from build123d import *

# Parameters (mm, degrees)
EXTRUDE_1_OUTLINE_R = 1.5
EXTRUDE_1_DEPTH     = 3
EXTRUDE_2_DEPTH     = 25
EXTRUDE_3_DEPTH     = 3
EXTRUDE_4_REACH     = 147.278
FILLET_1_R          = 3
SKETCH_5_R          = 1.5
CUT_EXTRUDE_3_DEPTH = 15
SKETCH_6_R          = 126.976740186
SKETCH_6_R_2        = 100
CUT_EXTRUDE_4_DEPTH = 30
SKETCH_8_W          = 28.33895888
SKETCH_8_H          = 14.242713356
CUT_EXTRUDE_5_DEPTH = 5


# Read off the part's stored shape, not the designer's step: 填料-伸長1
with BuildPart() as part:
    # 填料-伸長1 outline → 填料-伸長1 (new body)
    with BuildSketch(Plane.XZ.offset(-131.641882403)):
        with BuildLine():
            ThreePointArc((-105.458191259, 52.468420543), (-108.501205852, 56.151510861), (-113.143070085, 55.020940854))
            Line((-113.143070085, 55.020940854), (-129.654103506, 38.071506203))
            ThreePointArc((-129.654103506, 38.071506203), (-130.77342938, 33.752171981), (-127.62304878, 30.592323786))
            Line((-127.62304878, 30.592323786), (-107.96955265, 30.592323786))
            ThreePointArc((-107.96955265, 30.592323786), (-104.412306977, 32.020558846), (-103.246421534, 35.67221098))
            Line((-103.246421534, 35.67221098), (-105.458191259, 52.468420543))
        make_face()
        with Locations((-126.430709133, 34.931485706)):
            Circle(EXTRUDE_1_OUTLINE_R, mode=Mode.SUBTRACT)
        with Locations((-107.707905988, 35.084710794)):
            Circle(EXTRUDE_1_OUTLINE_R, mode=Mode.SUBTRACT)
        with Locations((-109.919675712, 51.880920357)):
            Circle(EXTRUDE_1_OUTLINE_R, mode=Mode.SUBTRACT)
    extrude(amount=EXTRUDE_1_DEPTH)

    # 草圖2 → 填料-伸長2 (add)
    with BuildSketch(Plane.XZ.offset(-128.641882403)):
        Polygon((-104.786745972, 47.369455849), (-124.786745972, 47.369455849), (-124.786745972, 44.369455849), (-104.786745972, 44.369455849), (-104.391697962, 44.369455849), align=None)
    extrude(amount=EXTRUDE_2_DEPTH)

    # 草圖3 → 填料-伸長3 (add)
    with BuildSketch(Plane(origin=(0, 128.641882403, 0), x_dir=(1, 0, 0), z_dir=(0, 1, 0))):
        Polygon((-124.786745972, -47.369455849), (-120.596647578, -47.369455849), (-123.519051852, -44.369455849), (-124.786745972, -44.369455849), align=None)
    extrude(amount=EXTRUDE_3_DEPTH)

    # 填料-伸長4: up to this face of the body (flat: up to its plane)
    extrude_4_end = Plane(part.part.faces().sort_by_distance((-115.187288505, 131.641882403, 40.896845269))[0])
    # 草圖4 → 填料-伸長4 (add, up to the picked face)
    with BuildSketch(Plane.XZ.offset(-103.641882403), mode=Mode.PRIVATE) as extrude_4_sk1:
        with BuildLine():
            Line((-104.786745972, 47.369455849), (-103.657869092, 38.796749367))
            Line((-103.657869092, 38.796749367), (-128.657869092, 38.796749367))
            ThreePointArc((-128.657869092, 38.796749367), (-125.290449125, 43.179472861), (-121.686031693, 47.369455849))
            Line((-121.686031693, 47.369455849), (-104.786745972, 47.369455849))
        make_face()
    extrude_4_tool1 = split(extrude(extrude_4_sk1.sketch, amount=-EXTRUDE_4_REACH, mode=Mode.PRIVATE), bisect_by=extrude_4_end, keep=Keep.BOTH, mode=Mode.PRIVATE)
    add(extrude_4_tool1.solids().sort_by(Axis((-114.856202, 103.641882, 42.808825), (0, 1, 0)))[0])

    # 圓角1
    # the kernel refuses this fillet: 3 mm, written as the material it takes off along each edge
    with BuildSketch(Plane(origin=(-128.657869092, 88.125757689, 38.796749367), x_dir=(1, 0, 0), z_dir=(0, 1, 0))) as fillet_1_piece_1:
        with BuildLine():
            CenterArc((6.112644238, -3), FILLET_1_R, 90, 129.509532044)
            ThreePointArc((3.798087984, -4.90861975), (1.860953441, -2.483782776), (0, 0))
            Line((0, 0), (6.112644238, 0))
        make_face()
    extrude(amount=40.516124714, mode=Mode.SUBTRACT)
    with BuildSketch(Plane(origin=(-128.657869092, 88.125757689, 38.796749367), x_dir=(1, 0, 0), z_dir=(0, 1, 0))) as fillet_1_piece_2_section:
        with BuildLine():
            CenterArc((6.112644238, -3), FILLET_1_R, 90, 129.509532044)
            ThreePointArc((3.798087984, -4.90861975), (1.860953441, -2.483782776), (0, 0))
            Line((0, 0), (6.112644238, 0))
        make_face()
    fillet_1_piece_2 = extrude(amount=56.032249428, mode=Mode.PRIVATE)
    fillet_1_piece_2 = split(fillet_1_piece_2, bisect_by=Plane(origin=(-126.052723455, 130.141882403, 41.768510156), z_dir=(-0.7163098605374205, 0, 0.6977823326058501)), keep=Keep.TOP, mode=Mode.PRIVATE)
    add(fillet_1_piece_2, mode=Mode.SUBTRACT)
    with BuildSketch(Plane(origin=(-103.657869092, 95.089515631, 38.796749367), x_dir=(-0.13055559688671156, 0, 0.9914409897323968), z_dir=(0, 1, 0))) as fillet_1_piece_3:
        with BuildLine():
            CenterArc((FILLET_1_R * 1.14031556955, -FILLET_1_R), FILLET_1_R, 90, 97.501699304)
            Line((FILLET_1_R * 0.148874579822, -FILLET_1_R * 1.13055559689), (0, 0))
            Line((0, 0), (FILLET_1_R * 1.14031556955, 0))
        make_face()
    extrude(amount=33.552366772, mode=Mode.SUBTRACT)

    # 草圖5 → 除料-伸長3 (cut)
    with BuildSketch(Plane.XZ.offset(-103.641882403)):
        with Locations(Location((-106.94667544, 41.72393279, 0), (0, 0, 270))):
            Circle(SKETCH_5_R)
        with Locations(Location((-122.44667544, 41.72393279, 0), (0, 0, 270))):
            Circle(SKETCH_5_R)
    extrude(amount=-CUT_EXTRUDE_3_DEPTH, mode=Mode.SUBTRACT)

    # 草圖6 → 除料-伸長4 (cut)
    with BuildSketch(Plane.XZ.offset(-103.641882403)):
        with Locations((-47.707905988, -19.915289206)):
            Circle(SKETCH_6_R)
        with Locations((-47.707905988, -19.915289206)):
            Circle(SKETCH_6_R_2, mode=Mode.SUBTRACT)
    extrude(amount=-CUT_EXTRUDE_4_DEPTH, mode=Mode.SUBTRACT)

    # 草圖8 → 除料-伸長5 (cut)
    with BuildSketch(Plane.XZ.offset(-103.641882403)):
        with Locations((-114.972608674, 43.454782353)):
            Rectangle(SKETCH_8_W, SKETCH_8_H)
    extrude(amount=-CUT_EXTRUDE_5_DEPTH, mode=Mode.SUBTRACT)


solid = part.part
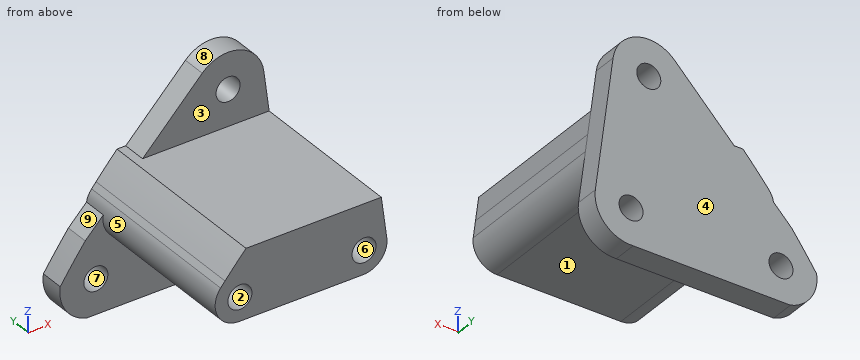
Input: part model. Units: mm. Frame: model coordinates. Face numbers are marked on the shaded views. A direction names the side the tool comes from. Round coordinates to 2 decimals unless told otherwise and drop trailing zeros. Order: outer loops, then holes, each group sorted by start corner. A loop starts at its lowest first (then second) coordinate and runs counter-clockwise, first axis right, second up.
1. Cut plane B-B, the plane x = -110. Output: boundary loops of the cut face in (y, z), then the cut area to 3 significant figures.
The answers:
outline: (108.64, 38.8) - (128.64, 38.8) - (128.64, 30.59) - (131.64, 30.59) - (131.64, 50.38) - (128.64, 50.38) - (128.64, 47.37) - (108.64, 47.37) - close; (128.64, 53.38) - (131.64, 53.38) - (131.64, 56.38) - (128.64, 56.38) - close
area: 240 mm2
2. Cut plane A-A, the plane y = 121. Output: boundary loops of the cut face in (x, z), then the cut area to 3 significant figures.
The answers:
outline: (-124.86, 43.71) arc R3 ccw to (-122.55, 38.8) - (-107.08, 38.8) arc R3 ccw to (-104.1, 42.19) - (-104.79, 47.37) - (-121.69, 47.37) arc R100 ccw to start
area: 170 mm2
3. Pin query (flat end, axial travel): P1, Ø5, axis at x = -126.43, z = 34.93, coming from the -Y side; P2, Ø5, axis at x = -120.5, y = 123.5, coming from the +Z side; P3, Ø10, axis at x = -125, z = 49.5, coming from the +Y side; P4, Ø1.5, axis at x = -119, y = 130.5, coming from the -Z side. Return the tip coordinate at first contact, or that it passes through.
The answers:
P1: stops at y = 128.64
P2: stops at z = 47.37
P3: stops at y = 131.64
P4: stops at z = 30.59
4. Set-up query: the marked faces 1, 2, 3, 4 and 5. Return all of +Z, -Z, +X, -X, +Y, -Y with unobstructed straight access to the full face (end or side cutting, diameter ignored); none if empty.
The answers:
face 1: -Z, +X, -X, -Y
face 2: -Y
face 3: +Z, +X, -X, -Y
face 4: +Z, -Z, +X, -X, +Y
face 5: -X, -Y
5. Material intervals for line 1 (Z direction, x = -120, y = 124); line 2 (Y direction, x = -129, z = 38.25); line 3 (Z direction, x = -121.5, y = 118.5), sorted ascending.
The answers:
line 1: z = 38.8 to 47.37
line 2: y = 128.64 to 131.64
line 3: z = 38.8 to 40.56, 42.89 to 47.37
6. Mould query, pull axis X, two halves, no side actions, for the marked faces 6, 7, 8 and 9. Classes: released by +X, released by -X, zero draft, split by the parting line, or undercut.
The answers:
face 6: undercut
face 7: undercut
face 8: split by the parting line
face 9: released by -X
7. Cut plane C-C, the plane y = 130.25. Output: boundary loops of the cut face in (x, z), then the cut area to 3 significant figures.
The answers:
outline: (-130.88, 35.6) arc R4.5 ccw to (-127.62, 30.59) - (-107.97, 30.59) arc R4.5 ccw to (-103.25, 35.67) - (-105.46, 52.47) arc R4.5 ccw to (-113.14, 55.02) - (-120.6, 47.37) - (-121.69, 47.37) arc R100 ccw to (-124.86, 43.71) arc R3 ccw to (-125.5, 42.34) - (-127.76, 40.02) arc R100 ccw to start; hole circle Ø3 at (-126.43, 34.93); hole circle Ø3 at (-109.92, 51.88); hole circle Ø3 at (-107.71, 35.08)
area: 468 mm2
8. Cut plane D-D, the plane z = 41. Output: boundary loops of the cut face in (x, y).
The answers:
outline: (-126.8, 128.64) - (-125.44, 128.64) - (-125.44, 108.64) - (-123.76, 108.64) - (-123.76, 118.64) - (-121.13, 118.64) - (-121.13, 108.64) - (-108.26, 108.64) - (-108.26, 118.64) - (-105.63, 118.64) - (-105.63, 108.64) - (-104.19, 108.64) - (-104.19, 128.64) - (-103.95, 128.64) - (-103.95, 131.64) - (-126.8, 131.64) - close
